```python
from build123d import *

# Parameters (mm, degrees)
F0_R     = 57
F1_DEPTH = 200
F2_T     = -2.5
F4_DEPTH = 60


with BuildPart() as f1:
    # F0 (on Top) → F1 (new body)
    with BuildSketch(Plane.XY):
        with Locations((0, 3.563962)):
            Circle(F0_R)
    extrude(amount=F1_DEPTH)

    # F2
    f2_openings = [f1.faces().sort_by_distance(p)[0] for p in [
        (0, 3.563962, 0),
        (0, 3.563962, 200),
    ]]
    offset(amount=F2_T, openings=f2_openings)

    # F3 (on Front) → F4 (cut, symmetric)
    with BuildSketch(Plane.XZ):
        Polygon((-57, 120.229874), (-57, 18.429874), (-18, 36.621924), align=None)
    extrude(amount=F4_DEPTH, both=True, mode=Mode.SUBTRACT)


solid = f1.part
```
Design review of the part built by this model. Coordinates are the model's own, in mm. A direction names the side the tool comes from. Give positions to 0.01 mm unless a question says otherwise; leave off trailing zeros. Order: outer loops, then holes, each group sorted by start corner. A loop starts at its lowest first (then second) coordinate and runs counter-clockwise, first axis right, second up. Notation, with made-up numbers: (-28, -3.75) - (-7, -3.75) arc R36 ccw to (-7, 30.25) - close; hole circle Ø1 at (22, 73). An arc over 180 degrees is marked (long way). Use a Markdown table: item, result. Add a question column.
(1) Add section B-B on y = 46.5. Give the boundary of the cut face in (x, z), then the cut area to 3 significant figures.
(2) Machinability: for faces 4 (the face through (-54.92, 3.31, 19.4)), 5 (the face through (51.983, 19.934, 98.6)), which of the approach directions +Z, -Z, +X, -X, +Y, -Y give a long, thin tool a straight path to every point of the face, cutting with its end or side? Answer none if there is none.
(3) Mouldability with a two-part tool opening along Z and no side actions: class faces 1 (the face through (46, -26, 200)), 2 (the face through (-47.52, 31.35, 99.91)), 3 (the face through (46, -26, 0)) as +Z half, -Z half, draft (parallel to the pull), parting line (faces both ways), or undercut.
(4) Add section A-A on x = 0. Give the boundary of the cut face in (y, z), then the cut area to 3 significant figures.
(5) Add section C-C on y = -20. Give the boundary of the cut face in (x, z), then the cut area to 3 significant figures.
(6) Clearance check with flat-ended pins moving along their axes: P1, Ø3, axis at x = -1, z = 133, coming from the +Y side; P2, Ø1, axis at y = -14.5, z = 126, coming from the -X side; P3, Ø3, axis at x = -44, z = 160, coming from the -Y side. State where each tip first meets the part, or that it passes through.
(7) Add section D-D on x = -14. Give the boundary of the cut face in (y, z).
(8) Wall thickness on probe 1 along Y at (x, z) = (0, 75.5); probe 2 along Y at (x, z) = (-9.5, 40); probe 3 along X at (y, z) = (-5.5, 161.5): over which ranges is each line inside the solid? List them lowest first. Write a range as [from, to].
Report:
| question | item | result |
|---|---|---|
| 1 | outline | (-37.49, 0) - (-33.57, 0) - (-33.57, 29.36) - (-37.49, 27.53) - close; (-37.49, 78.4) - (-33.57, 69.99) - (-33.57, 200) - (-37.49, 200) - close; (33.57, 0) - (37.49, 0) - (37.49, 200) - (33.57, 200) - close |
| 1 | area | 1,390 mm² |
| 2 | face 4 | -X, +Y, -Y |
| 2 | face 5 | +Z, -Z |
| 3 | face 1 | +Z half |
| 3 | face 2 | undercut |
| 3 | face 3 | -Z half |
| 4 | outline | (-53.44, 0) - (-50.94, 0) - (-50.94, 200) - (-53.44, 200) - close; (58.06, 0) - (60.56, 0) - (60.56, 200) - (58.06, 200) - close |
| 4 | area | 1,000 mm² |
| 5 | outline | (-51.9, 0) - (-49.14, 0) - (-49.14, 22.1) - (-51.9, 20.81) - close; (-51.9, 109.3) - (-49.14, 103.39) - (-49.14, 200) - (-51.9, 200) - close; (49.14, 0) - (51.9, 0) - (51.9, 200) - (49.14, 200) - close |
| 5 | area | 869 mm² |
| 6 | P1 | stops at y = 60.56 |
| 6 | P2 | stops at x = -54.23 |
| 6 | P3 | stops at y = -34.42 |
| 7 | outline | (-51.69, 0) - (-49.11, 0) - (-49.11, 200) - (-51.69, 200) - close; (56.24, 0) - (58.82, 0) - (58.82, 200) - (56.24, 200) - close |
| 8 | probe 1 | y = [-53.44, -50.94], [58.06, 60.56] |
| 8 | probe 2 | y = [-52.64, -50.1], [57.23, 59.77] |
| 8 | probe 3 | x = [-56.27, -53.74], [53.74, 56.27] |
